from build123d import *

# Parameters (mm, degrees)
SKETCH1_W           = 300
SKETCH1_H           = 140
SKETCH1_W_2         = 250
SKETCH1_H_2         = 90
BOSS_EXTRUDE1_DEPTH = 10
SKETCH2_W           = 30
SKETCH2_H           = 4
CUT_EXTRUDE1_DEPTH  = 44


with BuildPart() as part:
    # Sketch1 → Boss-Extrude1 (new body)
    with BuildSketch(Plane.XY):
        with Locations((125, 45)):
            Rectangle(SKETCH1_W, SKETCH1_H)
        with Locations((125, 45)):
            Rectangle(SKETCH1_W_2, SKETCH1_H_2, mode=Mode.SUBTRACT)
    extrude(amount=BOSS_EXTRUDE1_DEPTH)

    # Chamfer1
    # the kernel refuses this chamfer: 20, 11.547005384 mm, written as the material it takes off along each edge
    with BuildSketch(Plane(origin=(250, 0, 10), x_dir=(-0.05789386240267053, 0, -0.9983227437537926), z_dir=(0, 1, 0)), Plane(origin=(0, 90, 10), x_dir=(0.05789386240267081, 0, -0.9983227437537926), z_dir=(0, -1, 0))) as chamfer1_piece_1:
        with BuildLine():
            Line((11.967077239, 0), (-1.59731639, -20.634955616))
            Line((-1.59731639, -20.634955616), (-1.996645488, -20.611798071))
            ThreePointArc((-1.996645488, -20.611798071), (-0.998322744, -10.305899035), (-0.399329098, 0.023157545))
            Line((-0.399329098, 0.023157545), (0.023157545, 0.399329098))
            ThreePointArc((0.023157545, 0.399329098), (5.986641142, 0.053499955), (11.990234784, 0.399329098))
            Line((11.990234784, 0.399329098), (11.967077239, 0))
        make_face()
    extrude(amount=90, mode=Mode.SUBTRACT)
    with BuildSketch(Plane(origin=(250, 90, 10), x_dir=(0, -0.05789386240267053, -0.9983227437537926), z_dir=(-1, 0, 0)), Plane(origin=(0, 0, 10), x_dir=(0, 0.05789386240267081, -0.9983227437537926), z_dir=(1, 0, 0))) as chamfer1_piece_2:
        with BuildLine():
            Line((11.967077239, 0), (-1.59731639, -20.634955616))
            Line((-1.59731639, -20.634955616), (-1.996645488, -20.611798071))
            ThreePointArc((-1.996645488, -20.611798071), (-0.998322744, -10.305899035), (-0.399329098, 0.023157545))
            Line((-0.399329098, 0.023157545), (0.023157545, 0.399329098))
            ThreePointArc((0.023157545, 0.399329098), (5.986641142, 0.053499955), (11.990234784, 0.399329098))
            Line((11.990234784, 0.399329098), (11.967077239, 0))
        make_face()
    extrude(amount=250, mode=Mode.SUBTRACT)
    with BuildSketch(Plane(origin=(250, -51.741715093, 10), x_dir=(-0.05789386240267053, 0, -0.9983227437537926), z_dir=(0, 1, 0))) as chamfer1_piece_3a_section:
        with BuildLine():
            Line((11.967077239, 0), (-1.59731639, -20.634955616))
            Line((-1.59731639, -20.634955616), (-1.996645488, -20.611798071))
            ThreePointArc((-1.996645488, -20.611798071), (-0.998322744, -10.305899035), (-0.399329098, 0.023157545))
            Line((-0.399329098, 0.023157545), (0.023157545, 0.399329098))
            ThreePointArc((0.023157545, 0.399329098), (5.986641142, 0.053499955), (11.990234784, 0.399329098))
            Line((11.990234784, 0.399329098), (11.967077239, 0))
        make_face()
    chamfer1_piece_3a = extrude(amount=141.741715093, mode=Mode.PRIVATE)
    chamfer1_piece_3a = split(chamfer1_piece_3a, bisect_by=Plane(origin=(256.707645432, 0, 6.297222994), z_dir=(0, -1, 0)), keep=Keep.TOP, mode=Mode.PRIVATE)
    with BuildSketch(Plane(origin=(0, 0, 10), x_dir=(0, 0.05789386240267081, -0.9983227437537926), z_dir=(1, 0, 0))) as chamfer1_piece_3b_section:
        with BuildLine():
            Line((11.967077239, 0), (-1.59731639, -20.634955616))
            Line((-1.59731639, -20.634955616), (-1.996645488, -20.611798071))
            ThreePointArc((-1.996645488, -20.611798071), (-0.998322744, -10.305899035), (-0.399329098, 0.023157545))
            Line((-0.399329098, 0.023157545), (0.023157545, 0.399329098))
            ThreePointArc((0.023157545, 0.399329098), (5.986641142, 0.053499955), (11.990234784, 0.399329098))
            Line((11.990234784, 0.399329098), (11.967077239, 0))
        make_face()
    chamfer1_piece_3b = extrude(amount=301.741715093, mode=Mode.PRIVATE)
    chamfer1_piece_3b = split(chamfer1_piece_3b, bisect_by=Plane(origin=(250, -6.707645432, 6.297222994), z_dir=(1, 0, 0)), keep=Keep.TOP, mode=Mode.PRIVATE)
    chamfer1_piece_3 = chamfer1_piece_3a & chamfer1_piece_3b
    add(chamfer1_piece_3, mode=Mode.SUBTRACT)
    with BuildSketch(Plane(origin=(301.741715093, 90, 10), x_dir=(0, -0.05789386240267053, -0.9983227437537926), z_dir=(-1, 0, 0))) as chamfer1_piece_4a_section:
        with BuildLine():
            Line((11.967077239, 0), (-1.59731639, -20.634955616))
            Line((-1.59731639, -20.634955616), (-1.996645488, -20.611798071))
            ThreePointArc((-1.996645488, -20.611798071), (-0.998322744, -10.305899035), (-0.399329098, 0.023157545))
            Line((-0.399329098, 0.023157545), (0.023157545, 0.399329098))
            ThreePointArc((0.023157545, 0.399329098), (5.986641142, 0.053499955), (11.990234784, 0.399329098))
            Line((11.990234784, 0.399329098), (11.967077239, 0))
        make_face()
    chamfer1_piece_4a = extrude(amount=301.741715093, mode=Mode.PRIVATE)
    chamfer1_piece_4a = split(chamfer1_piece_4a, bisect_by=Plane(origin=(250, 96.707645432, 6.297222994), z_dir=(1, 0, 0)), keep=Keep.TOP, mode=Mode.PRIVATE)
    with BuildSketch(Plane(origin=(250, 0, 10), x_dir=(-0.05789386240267053, 0, -0.9983227437537926), z_dir=(0, 1, 0))) as chamfer1_piece_4b_section:
        with BuildLine():
            Line((11.967077239, 0), (-1.59731639, -20.634955616))
            Line((-1.59731639, -20.634955616), (-1.996645488, -20.611798071))
            ThreePointArc((-1.996645488, -20.611798071), (-0.998322744, -10.305899035), (-0.399329098, 0.023157545))
            Line((-0.399329098, 0.023157545), (0.023157545, 0.399329098))
            ThreePointArc((0.023157545, 0.399329098), (5.986641142, 0.053499955), (11.990234784, 0.399329098))
            Line((11.990234784, 0.399329098), (11.967077239, 0))
        make_face()
    chamfer1_piece_4b = extrude(amount=141.741715093, mode=Mode.PRIVATE)
    chamfer1_piece_4b = split(chamfer1_piece_4b, bisect_by=Plane(origin=(256.707645432, 90, 6.297222994), z_dir=(0, 1, 0)), keep=Keep.TOP, mode=Mode.PRIVATE)
    chamfer1_piece_4 = chamfer1_piece_4a & chamfer1_piece_4b
    add(chamfer1_piece_4, mode=Mode.SUBTRACT)
    with BuildSketch(Plane(origin=(0, 141.741715093, 10), x_dir=(0.05789386240267081, 0, -0.9983227437537926), z_dir=(0, -1, 0))) as chamfer1_piece_5a_section:
        with BuildLine():
            Line((11.967077239, 0), (-1.59731639, -20.634955616))
            Line((-1.59731639, -20.634955616), (-1.996645488, -20.611798071))
            ThreePointArc((-1.996645488, -20.611798071), (-0.998322744, -10.305899035), (-0.399329098, 0.023157545))
            Line((-0.399329098, 0.023157545), (0.023157545, 0.399329098))
            ThreePointArc((0.023157545, 0.399329098), (5.986641142, 0.053499955), (11.990234784, 0.399329098))
            Line((11.990234784, 0.399329098), (11.967077239, 0))
        make_face()
    chamfer1_piece_5a = extrude(amount=141.741715093, mode=Mode.PRIVATE)
    chamfer1_piece_5a = split(chamfer1_piece_5a, bisect_by=Plane(origin=(-6.707645432, 90, 6.297222994), z_dir=(0, 1, 0)), keep=Keep.TOP, mode=Mode.PRIVATE)
    with BuildSketch(Plane(origin=(250, 90, 10), x_dir=(0, -0.05789386240267053, -0.9983227437537926), z_dir=(-1, 0, 0))) as chamfer1_piece_5b_section:
        with BuildLine():
            Line((11.967077239, 0), (-1.59731639, -20.634955616))
            Line((-1.59731639, -20.634955616), (-1.996645488, -20.611798071))
            ThreePointArc((-1.996645488, -20.611798071), (-0.998322744, -10.305899035), (-0.399329098, 0.023157545))
            Line((-0.399329098, 0.023157545), (0.023157545, 0.399329098))
            ThreePointArc((0.023157545, 0.399329098), (5.986641142, 0.053499955), (11.990234784, 0.399329098))
            Line((11.990234784, 0.399329098), (11.967077239, 0))
        make_face()
    chamfer1_piece_5b = extrude(amount=301.741715093, mode=Mode.PRIVATE)
    chamfer1_piece_5b = split(chamfer1_piece_5b, bisect_by=Plane(origin=(0, 96.707645432, 6.297222994), z_dir=(-1, 0, 0)), keep=Keep.TOP, mode=Mode.PRIVATE)
    chamfer1_piece_5 = chamfer1_piece_5a & chamfer1_piece_5b
    add(chamfer1_piece_5, mode=Mode.SUBTRACT)
    with BuildSketch(Plane(origin=(0, 90, 10), x_dir=(0.05789386240267081, 0, -0.9983227437537926), z_dir=(0, -1, 0))) as chamfer1_piece_6a_section:
        with BuildLine():
            Line((11.967077239, 0), (-1.59731639, -20.634955616))
            Line((-1.59731639, -20.634955616), (-1.996645488, -20.611798071))
            ThreePointArc((-1.996645488, -20.611798071), (-0.998322744, -10.305899035), (-0.399329098, 0.023157545))
            Line((-0.399329098, 0.023157545), (0.023157545, 0.399329098))
            ThreePointArc((0.023157545, 0.399329098), (5.986641142, 0.053499955), (11.990234784, 0.399329098))
            Line((11.990234784, 0.399329098), (11.967077239, 0))
        make_face()
    chamfer1_piece_6a = extrude(amount=141.741715093, mode=Mode.PRIVATE)
    chamfer1_piece_6a = split(chamfer1_piece_6a, bisect_by=Plane(origin=(-6.707645432, 0, 6.297222994), z_dir=(0, -1, 0)), keep=Keep.TOP, mode=Mode.PRIVATE)
    with BuildSketch(Plane(origin=(-51.741715093, 0, 10), x_dir=(0, 0.05789386240267081, -0.9983227437537926), z_dir=(1, 0, 0))) as chamfer1_piece_6b_section:
        with BuildLine():
            Line((11.967077239, 0), (-1.59731639, -20.634955616))
            Line((-1.59731639, -20.634955616), (-1.996645488, -20.611798071))
            ThreePointArc((-1.996645488, -20.611798071), (-0.998322744, -10.305899035), (-0.399329098, 0.023157545))
            Line((-0.399329098, 0.023157545), (0.023157545, 0.399329098))
            ThreePointArc((0.023157545, 0.399329098), (5.986641142, 0.053499955), (11.990234784, 0.399329098))
            Line((11.990234784, 0.399329098), (11.967077239, 0))
        make_face()
    chamfer1_piece_6b = extrude(amount=301.741715093, mode=Mode.PRIVATE)
    chamfer1_piece_6b = split(chamfer1_piece_6b, bisect_by=Plane(origin=(0, -6.707645432, 6.297222994), z_dir=(-1, 0, 0)), keep=Keep.TOP, mode=Mode.PRIVATE)
    chamfer1_piece_6 = chamfer1_piece_6a & chamfer1_piece_6b
    add(chamfer1_piece_6, mode=Mode.SUBTRACT)

    # Sketch2 → Cut-Extrude1 (cut)
    with BuildSketch(Plane.XY.offset(10)):
        with Locations((125, -20)):
            Rectangle(SKETCH2_W, SKETCH2_H)
    extrude(amount=-CUT_EXTRUDE1_DEPTH, mode=Mode.SUBTRACT)


solid = part.part
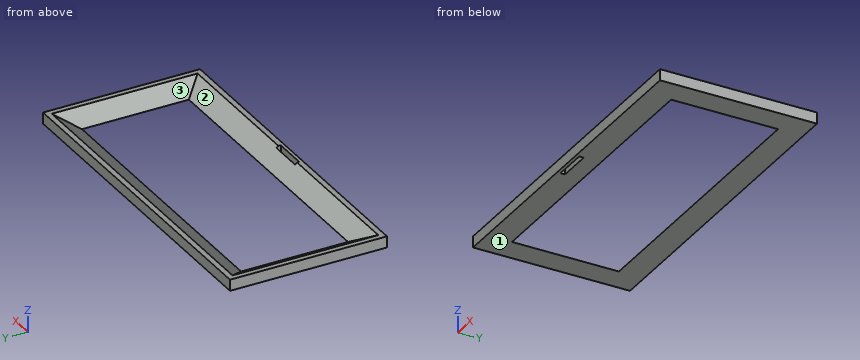
Build history of the part. All positions in model axes, mm. Face numbers are marked on the shaded views. Coordinates: 2 decimals unless noted, no trailing zeros. Order: outer loops, then holes, each group sorted by start corner. A loop starts at its lowest first (then second) coordinate and runs counter-clockwise, first axis right, second up. Notation, with made-up numbers: (-18, -22.75) - (8, -22.75) arc R18 ccw to (8, -17.75) - close; hole circle Ø6 at (57.5, 22.25). An arc over 180 degrees is marked (long way). Write item = value, one per line. Start each with the question number.
1) Saw through at D-D on y = 99. Write the cut outline in (x, z), then the cut area to 3 significant figures.
2) Two-plate mould, pull along X, no slides. Class the marked faces 1, 2 and 3: pulls with the +X half, pulls with the -X half, needs draft (parallel to the pull), parting line crosses it, or undercut.
3) Saw through at A-A on y = 56. Write the cut outline in (x, z), then the cut area to 3 significant figures.
4) Saw through at B-B on x = 206.5. Write the cut outline in (y, z).
5) Saw through at C-C on z = 4.5. Write the cut outline in (x, y).
6) Wall check: line 1 along Y through (x, z) = (112.5, 2.25); line 2 along Y through (x, z) = (147.5, 6.5); line 3 along Y through (x, z) = (160, 6.75). Give the ranges that are in metal, low to high. Write a range as from..to.
From the geometry:
q1.outline = (-25, 0) - (275, 0) - (275, 10) - (270, 10) - (259, 3.65) - (-9, 3.65) - (-20, 10) - (-25, 10) - close
q1.area = 1,230 mm^2
q2.face_1 = needs draft
q2.face_2 = undercut
q2.face_3 = undercut
q3.outline = (-25, 0) - (-2.68, 0) - (-20, 10) - (-25, 10) - close; (252.68, 0) - (275, 0) - (275, 10) - (270, 10) - close
q3.area = 273 mm^2
q4.outline = (-25, 0) - (-2.68, 0) - (-20, 10) - (-25, 10) - close; (92.68, 0) - (115, 0) - (115, 10) - (110, 10) - close
q5.outline = (-25, -25) - (275, -25) - (275, 115) - (-25, 115) - close; hole (-10.47, -10.47) - (260.47, -10.47) - (260.47, 100.47) - (-10.47, 100.47) - close; hole (110, -22) - (140, -22) - (140, -18) - (110, -18) - close
q6.line_1 = -25..-22, -18..-6.58, 96.58..115
q6.line_2 = -25..-13.94, 103.94..115
q6.line_3 = -25..-14.37, 104.37..115
